Job drawing, mm, ordinate dimensions from the low corner. One solid piece. A direction names the side the tool comes from. Give positions to 0.01 mm unless a question says otherwise; leave off trailing zeros. Order: outer loops, then holes, each group sorted by start corner. A loop starts at its lowest first (then second) coordinate and runs counter-clockwise, first axis right, second up. Notation, with made-up numbers: M 6.25,55.5 L 18.25,55.5 A16 cw 18.25,69.5 Z; hole C 54,5.25 d5. An arc over 180 degrees is marked long. Put each result on its own line as item: value. Start each with the question number.
1) Pin check, flat tips, straight feed: pin 1 (0.7 mm diameter, centred on x = 2, y = 7, fed in from +Z); pin 2 (1.6 mm diameter, centred on y = 8, z = 6, fed in from +X); pin 3 (0.7 mm diameter, centred on y = 7.5, z = 6, fed in from -X) (1 decimal). Stop position of each tip, or through.
2) Cut at C-C (y = 7.5). Write the cut outline in (x, z) (1 decimal).
3) Tool access for the marked faces 1, 2, 3, 4 and 5: list every direction of +Z, -Z, +X, -X, +Y, -Y with a clear straight run to the whole face (end or side of a thin tool).
4) Cut at B-B (x = 1.2). Write the cut outline in (y, z), and give its area (3 significant figures).
5) Drill centre lines: line 1 (Y direction, x = 0.45, z = 1.5); line 2 (Z direction, x = 2.3, y = 8). Where is each one in solid material? Low to high. Write a range as [from, to].
6) Cut at D-D (x = 2.85). Write the cut outline in (y, z).
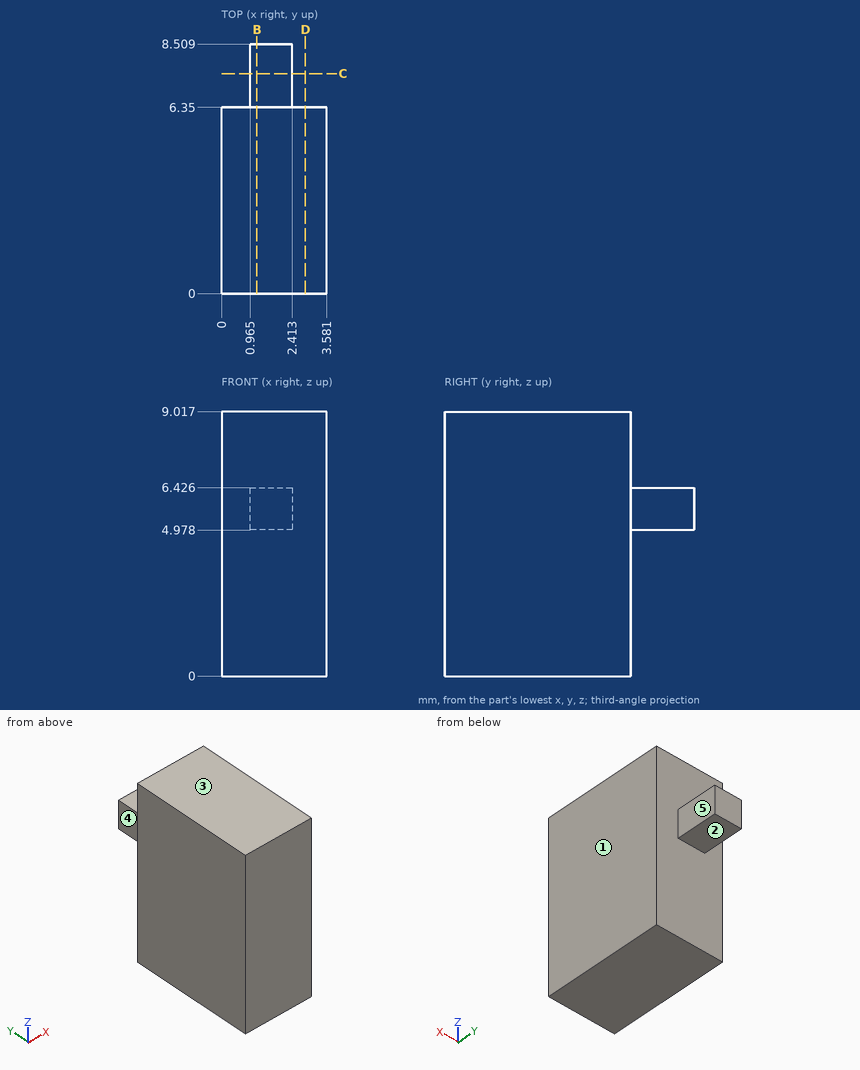
Solution:
1. pin 1: z = 6.43
1. pin 2: x = 2.41
1. pin 3: x = 1
2. outline: M 1,5 L 2.4,5 L 2.4,6.4 L 1,6.4 Z
3. face 1: +Z, -Z, +X, +Y, -Y
3. face 2: -Z, +X, -X, +Y
3. face 3: +Z, +X, -X, +Y, -Y
3. face 4: +Z, -Z, -X, +Y
3. face 5: +Z, -Z, +X, +Y
4. outline: M 0,0 L 6.35,0 L 6.35,4.98 L 8.51,4.98 L 8.51,6.43 L 6.35,6.43 L 6.35,9.02 L 0,9.02 Z
4. area: 60.4 mm²
5. line 1: [0, 6.35]
5. line 2: [4.98, 6.43]
6. outline: M 0,0 L 6.35,0 L 6.35,9.02 L 0,9.02 Z
